Read the model definition and answer for the solid it produces. Units are mm, in the model's axes. Face numbers are marked on the shaded views. A direction names the side the tool comes from. Give positions to 0.01 mm unless a question says otherwise; leave off trailing zeros. Write each loop counter-clockwise with the first axis right and the second up, starting at its lowest first coordinate (ties: lowest second). Pieces come first, ordered by that corner, then holes. Notation, with made-up numbers: (84, -37) -> (95, -37) arc R8 cw to (95, -22) -> close; hole circle Ø2 at (-11.5, 85.25). An arc over 180 degrees is marked (long way). Use a Markdown table: item, result.
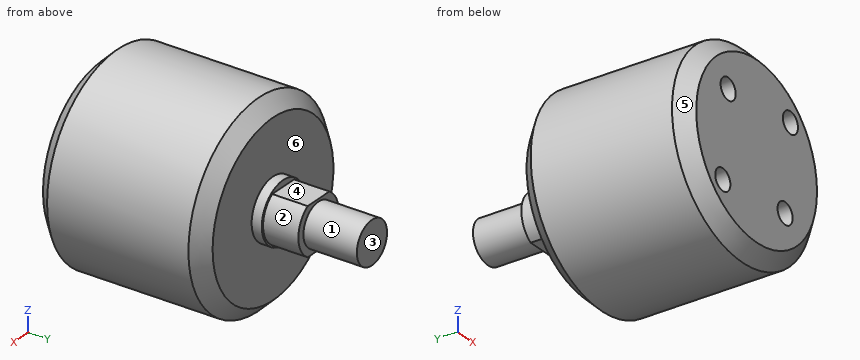
Autodesk Inventor part; units mm, degrees
ref_plane "YZ Plane" through (0, 0, 0) normal (1, 0, 0) x (0, 1, 0)
ref_plane "XZ Plane" through (0, 0, 0) normal (0, 1, 0) x (-1, 0, 0)
ref_plane "XY Plane" through (0, 0, 0) normal (0, 0, 1) x (1, 0, 0)
sketch "Sketch1" plane through (0, 0, 0) normal (0, 0, 1) x (1, 0, 0)
  line L0 (0, 0) -> (14, 0)
  line L1 (14, 0) -> (14, 24)
  line L2 (14, 24) -> (4.25, 24)
  line L3 (4.25, 24) -> (4.25, 25.4397)
  line L4 (4.25, 25.4397) -> (4, 25.4397)
  line L5 (3, 38) -> (0, 38)
  line L6 (0, 38) -> (0, 0)
  line L7 (4, 25.4397) -> (4, 30.4397)
  line L8 (4, 30.4397) -> (3, 30.4397)
  line L9 (3, 30.4397) -> (3, 38)
  dimension "d0" = 28
  dimension "d1" = 24
  dimension "d2" = 5
  dimension "d3" = 8
  dimension "d4" = 6
  dimension "d5" = 8.5
  dimension "d6" = 38
revolve "Revolution1" add sketch "Sketch1" angle 360 about axis through (0, 38, 0) along (0, -1, 0)
chamfer "Chamfer1" distance 2 angle 45 2 edges at (-14, 0, 0) (-14, 24, 0)
thread "Thread1"
sketch "Sketch2" plane through (0, 30.4397, 0) normal (0, 1, 0) x (1, 0, 0)
  line L0 (-2.1626, 3.365) -> (2.1626, 3.365)
  line L1 (2.1626, 3.365) -> (2.1626, -3.365)
  line L2 (2.1626, -3.365) -> (-2.1626, -3.365)
  line L3 (-2.1626, -3.365) -> (-2.1626, 3.365)
  circle A0 centre (0, 0) radius 3
  circle A1 centre (0, 0) radius 4
  point P0 (2.1626, 0)
  dimension "d13" = 6.73
extrude "Extrusion1" cut sketch "Sketch2" against normal blind 5 contours A1 L0 | L2 A1
sketch "Sketch4" plane through (0, 0, 0) normal (0, -1, 0) x (1, 0, 0)
  circle A0 centre (6.7175, 6.7175) radius 1.5
  circle A1 centre (-6.7175, -6.7175) radius 1.5
  circle A2 centre (-5.6569, 5.6569) radius 1.5
  circle A3 centre (5.6569, -5.6569) radius 1.5
  line L0 (-6.7175, -6.7175) -> (6.7175, 6.7175) construction
  line L1 (-5.6569, 5.6569) -> (5.6569, -5.6569) construction
  line L2 (0, 0) -> (0, 11.5514) construction
  point P0 (0, 0)
  dimension "d20" = 3
  dimension "d21" = 19
  dimension "d22" = 16
  dimension "d23" = 45
extrude "Extrusion3" cut sketch "Sketch4" against normal blind 5
properties part number "Unmodified Motor"
Item 1: A cutting plane is placed at D-D (y = 31). Give the vertices of the cut face in (x, z).
Return value:
| item | result |
|---|---|
| outline | circle Ø6 at (0, 0) |
Item 2: A cutting plane is placed at C-C (y = 23). Give the vertices of the cut face in (x, z).
Return value:
| item | result |
|---|---|
| outline | circle Ø26 at (0, 0) |
Item 3: A tool of negligible diameter and unlimited length cuts with its end or side. For the marked faces 1, 2 and 3, from which of +Z, -Z, +X, -X, +Y, -Y can it reach the whole face along a straight path? Write none if from no direction.
Return value:
| item | result |
|---|---|
| face 1 | +Y |
| face 2 | +X, +Y |
| face 3 | +Z, -Z, +X, -X, +Y |
Item 4: A cutting plane is placed at A-A (z = 0). Give the vertices of the cut face in (x, y), then the cut area to 3 significant figures.
Return value:
| item | result |
|---|---|
| outline | (-14, 2) -> (-12, 0) -> (12, 0) -> (14, 2) -> (14, 22) -> (12, 24) -> (4.25, 24) -> (4.25, 25.44) -> (4, 25.44) -> (4, 30.44) -> (3, 30.44) -> (3, 38) -> (-3, 38) -> (-3, 30.44) -> (-4, 30.44) -> (-4, 25.44) -> (-4.25, 25.44) -> (-4.25, 24) -> (-12, 24) -> (-14, 22) -> close |
| area | 762 mm^2 |
Item 5: Each of these flat-tipped pins is pushed along its axis until it touches: P1, Ø1.8, axis at x = -5.66, z = 5.66, coming from the +Y side; P2, Ø4, axis at x = 0.5, z = -5.5, coming from the +Y side; P3, Ø1, axis at y = 13.5, z = -9.5, coming from the +X side. Where does it stop, or does it pass through?
Return value:
| item | result |
|---|---|
| P1 | y = 24 |
| P2 | y = 25.44 |
| P3 | x = 10.72 |
Item 6: A cutting plane is placed at B-B (x = 0). Give the vertices of the cut face in (y, z) (3 decimals).
Return value:
| item | result |
|---|---|
| outline | (0, -12) -> (2, -14) -> (22, -14) -> (24, -12) -> (24, -4.25) -> (25.44, -4.25) -> (25.44, -3.365) -> (30.44, -3.365) -> (30.44, -3) -> (38, -3) -> (38, 3) -> (30.44, 3) -> (30.44, 3.365) -> (25.44, 3.365) -> (25.44, 4.25) -> (24, 4.25) -> (24, 12) -> (22, 14) -> (2, 14) -> (0, 12) -> close |
Item 7: For a pull along Y with two mould halves and no side action, classify the marked faces 4, 5 and 6 as +Y half, -Y half, draft (parallel to the pull), parting line (faces both ways), or undercut.
Return value:
| item | result |
|---|---|
| face 4 | draft |
| face 5 | -Y half |
| face 6 | +Y half |
Item 8: Straight lines are drawn through the part: line 1 along X through (y, z) = (4.5, -7); line 2 along Y through (x, z) = (7.5, 5.25); line 3 along Y through (x, z) = (0.5, -4). For each, find the intervals that lie inside material, in ascending order. Write a range as [from, to].
Return value:
| item | result |
|---|---|
| line 1 | [-12.12, -8.19], [-5.24, 4.99], [6.32, 12.12] |
| line 2 | [0, 24] |
| line 3 | [0, 25.44] |
